Geometry check sheet. Reference: the model listing, model coordinates, mm. Face numbers are marked on the shaded views. A direction names the side the tool comes from. Round coordinates to 2 decimals unless told otherwise and drop trailing zeros. Write each loop counter-clockwise with the first axis right and the second up, starting at its lowest first coordinate (ties: lowest second). Pieces come first, ordered by that corner, then holes. Notation, with made-up numbers: (51, 5) - (97, 5) arc R11 ccw to (97, 15) - close; hole circle Ø6 at (-40, 85). An arc over 180 degrees is marked (long way). Return JSON: item names as keys, results as strings. Group by question number.
Autodesk Inventor part; units mm, degrees
ref_plane "YZ Plane" through (0, 0, 0) normal (1, 0, 0) x (0, 1, 0)
ref_plane "XZ Plane" through (0, 0, 0) normal (0, 1, 0) x (-1, 0, 0)
ref_plane "XY Plane" through (0, 0, 0) normal (0, 0, 1) x (1, 0, 0)
sketch "Sketch1" plane through (0, 0, 0) normal (0, 0, 1) x (1, 0, 0)
  circle A0 centre (0, 0) radius 25
  circle A1 centre (0, 0) radius 30
  dimension "d0" = 50
  dimension "d1" = 60
extrude "Extrusion1" add sketch "Sketch1" along normal blind 20
sketch "Sketch2" plane through (0, 0, 20) normal (0, 0, 1) x (1, 0, 0)
  circle A0 centre (0, 0) radius 30
extrude "Extrusion2" add sketch "Sketch2" along normal blind 5
sketch "Sketch3" plane through (0, 0, 0) normal (0, 1, 0) x (-1, 0, 0)
  line L0 (30, 25) -> (-30, 25)
  arc A0 (-25, 25) -> (-10, 50) centre (-34.9158, 47.9495) ccw
  arc A1 (10, 50) -> (25, 25) centre (34.9158, 47.9495) ccw
  line L1 (-25, 20) -> (-25, 0)
  line L2 (25, 20) -> (25, 0)
  line L3 (-10, 50) -> (10, 50)
  arc A2 (-10, 50) -> (-23.3636, 64.782) centre (-26.3452, 48.6548) ccw construction
  line L4 (-10, 50) -> (-25, 65) construction
  line L5 (-10, 50) -> (11.2132, 50) construction
  arc A3 (23.3636, 64.782) -> (10, 50) centre (26.3452, 48.6548) ccw construction
  line L6 (-23, 75) -> (13, 75) construction
  line L7 (-25, 66.7486) -> (-25, 73) construction
  line L8 (25, 66.7486) -> (25, 73) construction
  arc A4 (-23, 75) -> (-25, 73) centre (-23, 73) ccw construction
  arc A5 (-25, 66.7486) -> (-23.3636, 64.782) centre (-23, 66.7486) ccw construction
  arc A6 (23.3636, 64.782) -> (25, 66.7486) centre (23, 66.7486) ccw construction
  arc A7 (25, 73) -> (23, 75) centre (23, 73) ccw construction
  line L9 (-13, 75) -> (15, 75)
  line L10 (15, 73) -> (15, 65.5675)
  line L11 (15, 65) -> (-15, 65) construction
  line L12 (-15, 65.5675) -> (-15, 73)
  arc A8 (-10, 50) -> (-14.7104, 64.531) centre (-43.196, 47.268) ccw
  arc A9 (14.7104, 64.531) -> (10, 50) centre (43.196, 47.268) ccw
  arc A10 (-15, 65.5675) -> (-14.7104, 64.531) centre (-13, 65.5675) ccw
  arc A11 (-13, 75) -> (-15, 73) centre (-13, 73) ccw
  arc A12 (15, 73) -> (13, 75) centre (13, 73) ccw
  arc A13 (14.7104, 64.531) -> (15, 65.5675) centre (13, 65.5675) ccw
  point P0 (0, 0)
  point P1 (25, 65)
  point P2 (-15, 75)
  dimension "d6" = 25
  dimension "d7" = 25
  dimension "d8" = 20
  dimension "d9" = 10
  dimension "d10" = 25
  dimension "d11" = 135
  dimension "d12" = 135
  dimension "d13" = 10
  dimension "d14" = 2
  dimension "d33" = 50
  dimension "d34" = 30
  dimension "d35" = 15
  dimension "d36" = 10
  dimension "d37" = 15
  dimension "d38" = 2
extrude "Extrusion3" add sketch "Sketch3" along normal mid plane 33
sketch "Sketch6" plane through (0, 0, 0) normal (1, 0, 0) x (0, 1, 0)
  line L0 (16.5, 25) -> (-16.5, 25)
  line L1 (16.5, 50) -> (-16.5, 50)
  line L2 (0, 50) -> (7.5, 50)
  line L3 (0, 50) -> (-7.5, 50)
  line L4 (-16.5, 25) -> (-16.5, 50)
  arc A0 (-16.5, 25) -> (-7.5, 50) centre (-47.499, 50.2796) ccw
  line L5 (16.5, 50) -> (16.5, 25)
  arc A1 (7.5, 50) -> (16.5, 25) centre (47.499, 50.2796) ccw
  line L6 (-16.5, 75) -> (16.5, 75)
  line L7 (10, 75) -> (-10, 75)
  line L8 (-10, 75) -> (-10, 65)
  line L9 (-10, 65) -> (10, 65)
  line L10 (10, 65) -> (10, 75)
  arc A2 (7.5, 50) -> (10, 65) centre (-36.25, 65) ccw
  arc A3 (-10, 65) -> (-7.5, 50) centre (36.25, 65) ccw
  line L11 (16.5, 64.531) -> (16.5, 50)
  line L12 (16.5, 50) -> (16.5, 75)
  line L13 (-16.5, 50) -> (-16.5, 64.531)
  line L14 (-16.5, 75) -> (-16.5, 50)
  point P0 (0, 0)
  dimension "d39" = 7.5
  dimension "d40" = 7.5
  dimension "d41" = 40
  dimension "d42" = 40
  dimension "d43" = 20
  dimension "d44" = 10
  dimension "d46" = 20
  dimension "d47" = 10
  dimension "d48" = 10
extrude "Extrusion6" cut sketch "Sketch6" along normal through all both and the other way through all contours A1 L1 L5 | L4 L1 A0 | L1 A2 L10 L6 L12 L11 | L13 L14 L6 L8 A3 L1
sketch "Sketch7" plane through (0, 0, 0) normal (0, 1, 0) x (-1, 0, 0)
  arc A0 (14.9178, 65) -> (15, 65.5675) centre (13, 65.5675) ccw
  line L0 (14.9178, 65) -> (-14.9178, 65)
  arc A1 (-15, 65.5675) -> (-14.9178, 65) centre (-13, 65.5675) ccw
  line L1 (-15, 73) -> (-15, 65.5675)
  arc A2 (-13, 75) -> (-15, 73) centre (-13, 73) ccw
  line L2 (13, 75) -> (-13, 75)
  arc A3 (15, 73) -> (13, 75) centre (13, 73) ccw
  line L3 (15, 65.5675) -> (15, 73)
  circle A4 centre (10, 70) radius 3
  circle A5 centre (-10, 70) radius 3
  point P0 (0, 0)
  dimension "d51" = 6
  dimension "d52" = 6
  dimension "d53" = 5
  dimension "d54" = 5
  dimension "d55" = 5
  dimension "d56" = 5
extrude "Extrusion7" cut sketch "Sketch7" along normal mid plane 12
properties part number "Arm 6 v0.1"
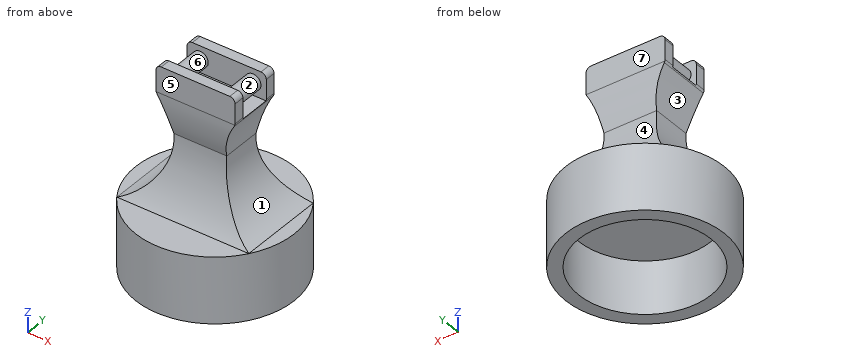
1. Mould release check, pull along Y, two halves, no side actions. Record for the marked faces 5, 6 and 7: pulls with the +Y half, pulls with the -Y half, needs draft (parallel to the pull), parting line crosses it, or undercut.
2. Material ranges on line 1 along Y through (x, z) = (0, 7); line 2 along Y through (x, z) = (4, 12.5); line 3 along Z through (x, y) = (-4.5, -1.5), recorded low to high.
3. Tool access check on the marked faces 1, 2, 3 and 4. Record the directions out of +Z, -Z, +X, -X, +Y, -Y that give a thin tool (end or side, any length) a straight path to the whole face; none if there is none.
4. Section check D-D (x = -8.5). Enter the section's corners in (y, z).
5. Section check A-A (y = 0). Enter the section's corners in (x, z), and give its area (3 significant figures).
6. Depth check by flat-ended pin: pin 1 Ø25 at (x, y) = (2, 9.5) entering from -Z; pin 2 Ø4.5 at (y, z) = (-8, 68) entering from +X; pin 3 Ø11 at (x, z) = (6, 71.5) entering from +Y. Enter the tip coordinate at first touch or a pass-through.
7. Section check B-B (z = 70). Enter the section's corners in (x, y).
8. Section check C-C (x = 0). Enter the section's corners in (y, z).
Result sheet:
{
 "1": {"face 5": "pulls with the -Y half", "face 6": "undercut", "face 7": "pulls with the +Y half"},
 "2": {"line 1": "y = -30 to -25, 25 to 30", "line 2": "y = -29.73 to -24.68, 24.68 to 29.73", "line 3": "z = 20 to 65"},
 "3": {"face 1": "+X, +Y, -Y", "face 2": "none", "face 3": "-X, +Y, -Y", "face 4": "+X, -X, +Y"},
 "4": {"outline": "(-28.77, 0) - (-23.51, 0) - (-23.51, 20) - (23.51, 20) - (23.51, 0) - (28.77, 0) - (28.77, 25) - (16.5, 25) arc R40 cw to (7.5, 50) arc R46.25 ccw to (10, 65) - (10, 75) - (6, 75) - (6, 72.6) - (-6, 72.6) - (-6, 75) - (-10, 75) - (-10, 65) arc R46.25 ccw to (-7.5, 50) arc R40 cw to (-16.5, 25) - (-28.77, 25) - close; hole (-6, 65) - (6, 65) - (6, 67.4) - (-6, 67.4) - close"},
 "5": {"outline": "(-30, 0) - (-25, 0) - (-25, 20) - (25, 20) - (25, 0) - (30, 0) - (30, 25) - (25, 25) arc R25 cw to (10, 50) arc R33.31 cw to (14.71, 64.53) arc R2 ccw to (14.92, 65) - (-14.92, 65) arc R2 ccw to (-14.71, 64.53) arc R33.31 cw to (-10, 50) arc R25 cw to (-25, 25) - (-30, 25) - close; circle Ø6 at (-10, 70); circle Ø6 at (10, 70)", "area": "1,600 mm²"},
 "6": {"pin 1": "stops at z = 20", "pin 2": "stops at x = 15", "pin 3": "stops at y = 10"},
 "7": {"outline": "(-15, -10) - (15, -10) - (15, -6) - (13, -6) - (13, 6) - (15, 6) - (15, 10) - (-15, 10) - (-15, 6) - (-13, 6) - (-13, -6) - (-15, -6) - close; hole (-7, -6) - (7, -6) - (7, 6) - (-7, 6) - close"},
 "8": {"outline": "(-30, 0) - (-25, 0) - (-25, 20) - (25, 20) - (25, 0) - (30, 0) - (30, 25) - (16.5, 25) arc R40 cw to (7.5, 50) arc R46.25 ccw to (10, 65) - (10, 75) - (6, 75) - (6, 65) - (-6, 65) - (-6, 75) - (-10, 75) - (-10, 65) arc R46.25 ccw to (-7.5, 50) arc R40 cw to (-16.5, 25) - (-30, 25) - close"}
}
